For this review, use the dimensioned drawing (mm, ordinates from the lowest corner) and the shaded views. Round coordinates to 2 decimals unless told otherwise and drop trailing zeros. Order: outer loops, then holes, each group sorted by start corner. A loop starts at its lowest first (then second) coordinate and runs counter-clockwise, first axis right, second up. Notation, with made-up numbers: M -33,-35.75 L -16,-35.75 A17 ccw -16,-17.75 Z; hole C 65,32 d7. An arc over 180 degrees is marked long. Put each result on its own line as item: value.
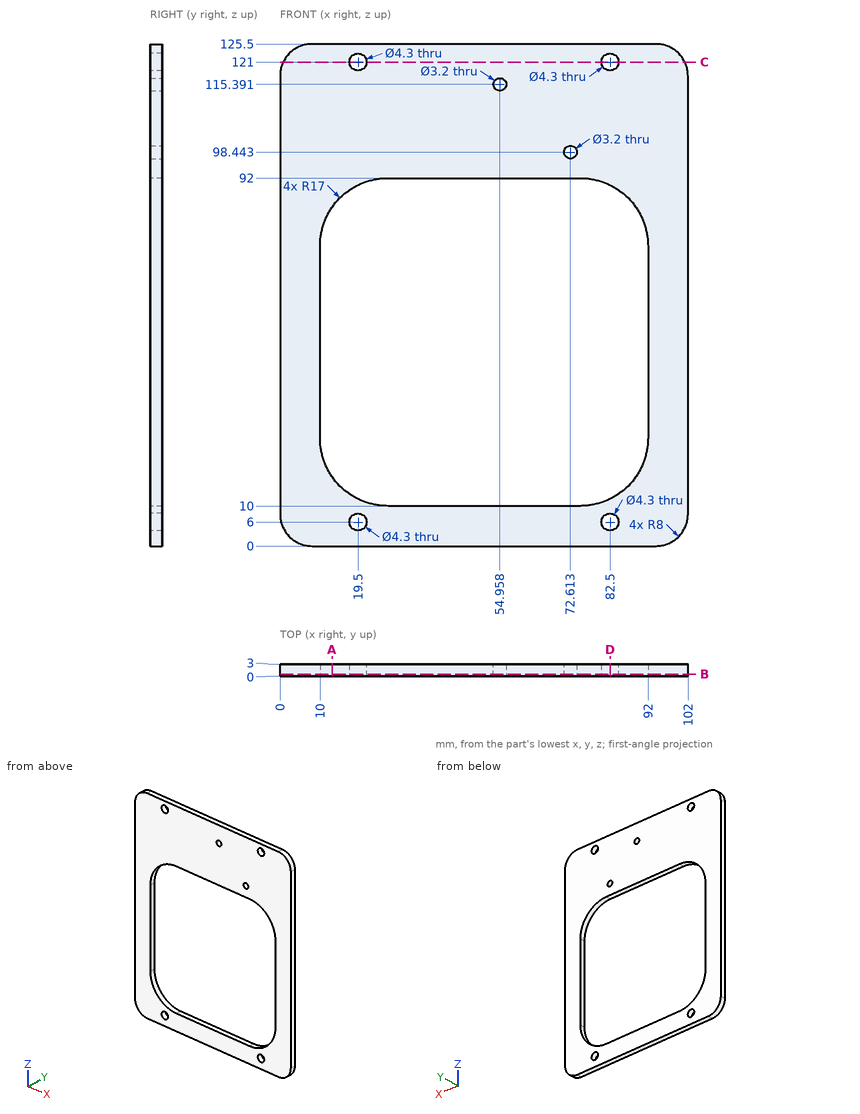
(1) Add section C-C on z = 121. Give the boundary of the cut face in (x, y).
A:
outline: M 0.81,0 L 17.35,0 L 17.35,3 L 0.81,3 Z; M 21.65,0 L 80.35,0 L 80.35,3 L 21.65,3 Z; M 84.65,0 L 101.19,0 L 101.19,3 L 84.65,3 Z
(2) Add section A-A on x = 13. Give the boundary of the cut face in (y, z), then the cut area to 3 significant figures.
A:
outline: M 0,0 L 3,0 L 3,17.36 L 0,17.36 Z; M 0,84.64 L 3,84.64 L 3,125.5 L 0,125.5 Z
area: 175 mm2
(3) To check wall thickness, follow L1, parallel to Z at x = 55, y = 2.2; L2, parallel to Z at x = 40.5, y = 1.4; L3, parallel to X at y = 1.9, z = 35. State the ranges of each line that lie inside material, in increasing order.
A:
L1: z = 0 to 10, 92 to 113.79, 116.99 to 125.5
L2: z = 0 to 10, 92 to 125.5
L3: x = 0 to 10, 92 to 102
(4) Add section D-D on x = 82.5. Give the boundary of the cut face in (y, z), then the cut area to 3 significant figures.
A:
outline: M 0,0 L 3,0 L 3,3.85 L 0,3.85 Z; M 0,8.15 L 3,8.15 L 3,11.74 L 0,11.74 Z; M 0,90.26 L 3,90.26 L 3,118.85 L 0,118.85 Z; M 0,123.15 L 3,123.15 L 3,125.5 L 0,125.5 Z
area: 115 mm2
(5) Add section B-B on y = 0.5. Give the boundary of the cut face in (x, z).
A:
outline: M 0,8 A8 ccw 8,0 L 94,0 A8 ccw 102,8 L 102,117.5 A8 ccw 94,125.5 L 8,125.5 A8 ccw 0,117.5 Z; hole M 10,27 A17 ccw 27,10 L 75,10 A17 ccw 92,27 L 92,75 A17 ccw 75,92 L 27,92 A17 ccw 10,75 Z; hole C 19.5,6 d4.3; hole C 19.5,121 d4.3; hole C 54.96,115.39 d3.2; hole C 72.61,98.44 d3.2; hole C 82.5,6 d4.3; hole C 82.5,121 d4.3
(6) Insertion check: pin 1 Ø1 at (y, z) = (1, 92) entering from -X; pin 2 Ø3 at (x, z) = (72.61, 98.44) entering from +Y. Each pin has a flat end and moves straight along its axis. Give the tip position at first contact, or say it passes through.
A:
pin 1: stops at x = 0
pin 2: passes through
